from build123d import *

# Parameters (mm, degrees)
SKETCH1_W               = 150
SKETCH1_H               = 100
BOSS_EXTRUDE1_DEPTH     = 50
SKETCH3_R               = 10
CUT_EXTRUDE1_DEPTH      = 100
SKETCH4_W               = 48
SKETCH4_H               = 30
CUT_EXTRUDE2_DEPTH      = 100
CUT_EXTRUDE3_DEPTH      = 112.130553854
CUT_EXTRUDE3_DEPTH_BACK = 112.130553854
SKETCH5_R               = 5


with BuildPart() as part:
    # Sketch1 → Boss-Extrude1 (new body)
    with BuildSketch(Plane(origin=(0, 0, 0), x_dir=(1, 0, 0), z_dir=(0, 1, 0))):
        Rectangle(SKETCH1_W, SKETCH1_H)
    extrude(amount=BOSS_EXTRUDE1_DEPTH)

    # Sketch3 → Cut-Extrude1 (cut)
    with BuildSketch(Plane.XY.offset(50)):
        with Locations((-40, 12)):
            Circle(SKETCH3_R)
    extrude(amount=-CUT_EXTRUDE1_DEPTH, mode=Mode.SUBTRACT)

    # Sketch4 → Cut-Extrude2 (cut)
    with BuildSketch(Plane.XZ):
        with Locations((44, 0)):
            Rectangle(SKETCH4_W, SKETCH4_H)
    extrude(amount=-CUT_EXTRUDE2_DEPTH, mode=Mode.SUBTRACT)

    # Sketch5 → Cut-Extrude3 (cut, two sides: drawn at the far end of the back side and taken through both)
    with BuildSketch(Plane(origin=(0, 0, 15), x_dir=(-1, 0, 0), z_dir=(0, 0, -1)).offset(-CUT_EXTRUDE3_DEPTH_BACK)):
        with Locations((-44, 7)):
            Circle(SKETCH5_R)
    extrude(amount=CUT_EXTRUDE3_DEPTH + CUT_EXTRUDE3_DEPTH_BACK, mode=Mode.SUBTRACT)


solid = part.part
Could you check a few things on this model? Use its own coordinates, in mm. A direction names the side the tool comes from. Coordinates: 2 decimals unless noted, no trailing zeros. Order: outer loops, then holes, each group sorted by start corner. A loop starts at its lowest first (then second) coordinate and runs counter-clockwise, first axis right, second up. Notation, with made-up numbers: (2, -10) -> (45, -10) arc R20 cw to (45, 12) -> close; hole circle Ø10 at (5.5, 81.25). An arc over 180 degrees is marked (long way). One line per question, with ' | ' between items.
Q1. If I drill on L1, parallel to X at y = 12.5, z = 3.5; L2, parallel to Y at x = 44, z = -24; L3, parallel to Z at x = 39.5, y = 33.5, over which ranges is the centre line in solid material (lowest first)?
Return value:
L1: -75 to -49.99, -30.01 to 20, 68 to 75 | L2: 0 to 2, 12 to 50 | L3: -50 to -15, 15 to 50
Q2. Imagine slicing it at B-B on z = -6. Please give me the cut outline in (x, y).
Return value:
outline: (-75, 0) -> (20, 0) -> (20, 50) -> (-75, 50) -> close; (68, 0) -> (75, 0) -> (75, 50) -> (68, 50) -> close; hole circle Ø20 at (-40, 12)
Q3. Thinking about a two-plate mould opening in X: for faces 1 (the face through (-1, 25, 50)), 2 (the face through (49, 7, -32)), 3 (the face through (75, 25, 1)), which applies, pulls with the +X half, pulls with the -X half, needs draft (parallel to the pull), parting line crosses it, or undercut?
Return value:
face 1: needs draft | face 2: undercut | face 3: pulls with the +X half
Q4. On a 3-axis mill with a long thin cutter (end or side, diameter ignored), from which of +Z, -Z, +X, -X, +Y, -Y can I reach the whole of each face in a straight line? I mean faces 4 (the face through (44, 25, -15)), 5 (the face through (-1, 50, -1)). Say none if no direction works.
Return value:
face 4: +Y, -Y | face 5: +Z, -Z, +X, -X, +Y
Q5. Imagine slicing it at C-C on x = 44. Please give me the cut outline in (y, z), and give its area (3 significant figures).
Return value:
outline: (0, -50) -> (2, -50) -> (2, -15) -> (0, -15) -> close; (0, 15) -> (2, 15) -> (2, 50) -> (0, 50) -> close; (12, -50) -> (50, -50) -> (50, -15) -> (12, -15) -> close; (12, 15) -> (50, 15) -> (50, 50) -> (12, 50) -> close | area: 2,800 mm²
Q6. I'm going to push flat-ended pins straight in: P1, Ø16, axis at x = -40, y = 12, coming from the -Z side; P2, Ø5, axis at x = -31.5, z = 10, coming from the -Y side. Where does each tip first touch, or does it pass through?
Return value:
P1: through | P2: y = 0
Q7. Imagine slicing it at D-D on x = -40. Please give me the cut outline in (y, z), and give its area (3 significant figures).
Return value:
outline: (0, -50) -> (2, -50) -> (2, 50) -> (0, 50) -> close; (22, -50) -> (50, -50) -> (50, 50) -> (22, 50) -> close | area: 3,000 mm²
Q8. Imagine slicing it at A-A on y = 20. Please give me the cut outline in (x, z), and give its area (3 significant figures).
Return value:
outline: (-75, -50) -> (-46, -50) -> (-46, 50) -> (-75, 50) -> close; (-34, -50) -> (75, -50) -> (75, 50) -> (-34, 50) -> close; hole (20, -15) -> (68, -15) -> (68, 15) -> (20, 15) -> close | area: 12,400 mm²
